Here's how the part is built. I have some questions about the finished solid (model axes, mm). Round coordinates to 2 decimals unless told otherwise and drop trailing zeros. Order: outer loops, then holes, each group sorted by start corner. A loop starts at its lowest first (then second) coordinate and runs counter-clockwise, first axis right, second up. Notation, with made-up numbers: (13.25, 57) -> (57.25, 57) arc R21 cw to (57.25, 71) -> close; hole circle Ø5 at (-17.75, 74.25). An arc over 180 degrees is marked (long way). Use a Markdown table: item, result. Add a question column.
from build123d import *

# Parameters (mm, degrees)
F1_DEPTH = 6.35
F4_R     = 6.1144864015
F5_DEPTH = 6.351


# Not quite as in the source:
# - the program builds the solid bodies; features that only make, move or delete a surface that nothing else refers to are left out


with BuildPart() as f1:
    # F0 (on Top) → F1 (new body)
    with BuildSketch(Plane.XY):
        Polygon((37.8358727575, 13.8656235676), (34.8533205688, 20.2251039445), (30.8117678713, 25.9700547725), (25.8340151985, 30.9259186276), (20.0713090466, 34.9421140946), (13.6987463258, 37.8966111063), (6.9099541298, 39.6996387661), (-0.0887935258, 40.2964129911), (-7.084843235, 39.6688010983), (-13.8656235676, 37.8358727575), (-20.2251039445, 34.8533205688), (-25.9700547725, 30.8117678713), (-30.9259186276, 25.8340151985), (-34.9421140946, 20.0713090466), (-37.8966111063, 13.6987463258), (-39.6996387661, 6.9099541298), (-40.2964129911, -0.0887935258), (-39.6688010983, -7.084843235), (-37.8358727575, -13.8656235676), (-34.8533205688, -20.2251039445), (-30.8117678713, -25.9700547725), (-25.8340151985, -30.9259186276), (-20.0713090466, -34.9421140946), (-13.6987463258, -37.8966111063), (-6.9099541298, -39.6996387661), (0.0887935258, -40.2964129911), (7.084843235, -39.6688010983), (13.8656235676, -37.8358727575), (20.2251039445, -34.8533205688), (25.9700547725, -30.8117678713), (30.9259186276, -25.8340151985), (34.9421140946, -20.0713090466), (37.8966111063, -13.6987463258), (39.6996387661, -6.9099541298), (40.2964129911, 0.0887935258), (39.6688010983, 7.084843235), align=None)
    extrude(amount=F1_DEPTH)

    # F4 (on face) → F5 (cut, through all)
    with BuildSketch(Plane.XY.offset(6.35)):
        with Locations((0, 28.4479867001)):
            Circle(F4_R)
    extrude(amount=-F5_DEPTH, mode=Mode.SUBTRACT)


solid = f1.part
(1) Please list where these lines run through material, in increasing order: probe 1 along Y at (x, z) = (0, 5); probe 2 along Y at (x, z) = (-4, 4); probe 3 along X at (y, z) = (28.5, 3.5). Write a range as from..to.
(2) I'm going to push flat-ended pins straight in: P1, Ø14, axis at x = 0, y = 28.45, coming from the +Z side; P2, Ø2, axis at y = 12, z = 4, coming from the +X side. Where does each tip first touch, or does it pass through?
(3) I want a section at C-C on y = 11.5. List the corners of the cut face in (x, z) for me, and give its area (3 significant figures).
(4) I want a section at B-B on x = 22. List the corners of the cut face in (y, z) for me, and give its area (3 significant figures).
(5) I want a section at A-A on x = 3. List the corners of the cut face in (y, z) for me.
Output:
| question | item | result |
|---|---|---|
| 1 | probe 1 | -40.29..22.33, 34.56..40.29 |
| 1 | probe 2 | -39.95..23.82, 33.07..39.95 |
| 1 | probe 3 | -28.27..-6.11, 6.11..28.27 |
| 2 | P1 | z = 6.35 |
| 2 | P2 | x = 38.61 |
| 3 | outline | (-38.48, 0) -> (38.48, 0) -> (38.48, 6.35) -> (-38.48, 6.35) -> close |
| 3 | area | 489 mm² |
| 4 | outline | (-33.6, 0) -> (33.6, 0) -> (33.6, 6.35) -> (-33.6, 6.35) -> close |
| 4 | area | 427 mm² |
| 5 | outline | (-40.04, 0) -> (23.12, 0) -> (23.12, 6.35) -> (-40.04, 6.35) -> close; (33.78, 0) -> (40.03, 0) -> (40.03, 6.35) -> (33.78, 6.35) -> close |
